Autodesk Inventor part; units mm, degrees
ref_plane "YZ Plane" through (0, 0, 0) normal (1, 0, 0) x (0, 1, 0)
ref_plane "XZ Plane" through (0, 0, 0) normal (0, 1, 0) x (-1, 0, 0)
ref_plane "XY Plane" through (0, 0, 0) normal (0, 0, 1) x (1, 0, 0)
sketch "Sketch1" plane through (0, 0, 0) normal (0, 1, 0) x (-1, 0, 0)
  arc A0 (16.9801, 0.913) -> (16.9801, -0.913) centre (-4, 0) ccw
  circle A1 centre (-4, 0) radius 21
  circle A2 centre (-4, 0) radius 19.1
  line L0 (17, 0) -> (25, 0)
  line L1 (25, 0) -> (25, -1.5)
  line L2 (25, -1.5) -> (15.041, -1.5)
  line L3 (25, 0) -> (25, 1.5)
  line L4 (25, 1.5) -> (15.041, 1.5)
  line L5 (25, -1.5) -> (25, -3)
  line L6 (25, -3) -> (14.8629, -3)
  line L7 (25, 1.5) -> (25, 3)
  line L8 (25, 3) -> (14.8629, 3)
  line L9 (-25, 0) -> (-34, 0)
  line L10 (-34, 0) -> (-42, 0)
  line L11 (-42, 0) -> (-42, 27.5)
  line L12 (-42, 27.5) -> (-34, 27.5)
  line L13 (-34, 27.5) -> (-34, 0)
  line L14 (-42, 0) -> (-42, -27.5)
  line L15 (-42, -27.5) -> (-34, -27.5)
  line L16 (-34, -27.5) -> (-34, 0)
  line L17 (-29.5, 0) -> (-29.5, 3)
  line L18 (-29.5, 3) -> (-24.7846, 3)
  line L19 (-29.5, 3) -> (-34, 3)
  line L20 (-29.5, 0) -> (-29.5, -3)
  line L21 (-29.5, -3) -> (-24.7846, -3)
  line L22 (-29.5, -3) -> (-34, -3)
  point P0 (-22.9783, -26)
  point P1 (16.7846, 3)
  point P2 (16.7846, -3)
  point P3 (-24.7846, 3)
  dimension "d8" = 38.2
  dimension "d9" = 8
  dimension "d10" = 1.5
  dimension "d11" = 1.5
  dimension "d12" = 1.5
  dimension "d13" = 1.5
  dimension "d31" = 21
  dimension "d60" = 9
  dimension "d61" = 8
  dimension "d62" = 27.5
  dimension "d63" = 27.5
  dimension "d64" = 3
  dimension "d65" = 3
extrude "Extrusion1" add sketch "Sketch1" along normal blind 23 contours A0 L8 A2 L6 | A0 L9 L17 L18 | A0 L21 L20 L9 | L8 L7 L4 A0 | A0 L4 A2 L8 | L17 L9 L13 L19 | L20 L22 L16 L9 | L13 L10 L11 L12 | L6 A2 L2 A0 | A0 L2 L5 L6 | L16 L15 L14 L10
sketch "Sketch4" plane through (-16.7846, 0, -3) normal (0, 0, -1) x (-1, 0, 0)
  line L0 (0, 0) -> (-41.5692, 0)
  line L1 (8.2154, 0) -> (8.2154, 23)
  line L2 (0, 0) -> (8.2154, 0)
  line L3 (8.2154, 0) -> (8.2154, 23)
  line L4 (8.2154, 23) -> (0, 23)
  line L5 (0, 23) -> (0, 0)
  line L6 (0, 11.5) -> (8.2154, 11.5)
  line L7 (4.1077, 11.5) -> (4.1077, 23)
  line L8 (4.1077, 11.5) -> (4.1077, 0)
  point P0 (-16.7846, 0)
  point P1 (4.1077, 5.75)
  point P2 (4.1077, 17.25)
hole "Hole2" at (-20.8923, 5.75, -3) at (-20.8923, 17.25, -3) direction (0, 0, 1) diameter 4 depth 8 tip angle 118
sketch "Sketch8" plane through (0, 23, 0) normal (0, 1, 0) x (1, 0, 0)
  line L0 (34, 3) -> (24.7846, 3)
  line L1 (34, 3) -> (24.7846, 3)
  line L2 (34, 27.5) -> (34, 3)
  line L3 (34, 3) -> (34, 27.5)
  line L4 (42, -27.5) -> (42, 27.5)
  line L5 (34, 27.5) -> (42, 27.5)
  line L6 (42, 27.5) -> (42, -27.5)
  line L7 (42, -27.5) -> (34, -27.5)
  line L8 (24.7846, -3) -> (34, -3)
  line L9 (34, -27.5) -> (34, -3)
  line L10 (34, -3) -> (24.7846, -3)
  arc A0 (24.7846, 3) -> (-16.7846, 3) centre (4, 0) ccw
  line L11 (4, 21) -> (4, 0)
  circle A1 centre (4, 0) radius 21
  point P0 (0, 0)
  point P1 (24.7846, 3)
  point P2 (24.7846, -3)
  dimension "d78" = 42
extrude "Extrusion5" cut sketch "Sketch8" against normal blind 19.5 contours L2 L5 L4 L7 L9 L8 A1 L0
sketch "Sketch9" plane through (0, 3.5, 0) normal (0, 1, 0) x (1, 0, 0)
  line L0 (34, 3) -> (34, 27.5)
  line L1 (34, -3) -> (34, 3)
  line L2 (34, 3) -> (34, 0)
  line L3 (42, 27.5) -> (42, -27.5)
  line L4 (42, 0) -> (34, 0)
  line L5 (38, 0) -> (38, -22.5)
  line L6 (38, 0) -> (38, 22.5)
  point P0 (0, 0)
  dimension "d69" = 22.5
  dimension "d70" = 22.5
hole "Hole4" at (38, 3.5, -22.5) at (38, 3.5, 22.5) direction (0, -1, 0) diameter 3 depth 8 tip angle 118
properties part number "Bracket kamera"
Verification items for the finished model (mm, model axes). A direction names the side the tool comes from. Coordinates: 2 decimals unless noted, no trailing zeros. Loops run counter-clockwise (first coordinate to the right, second up) from the corner with the lowest first, then second, coordinate; pieces in that order, holes last. Notation, with made-up numbers: (-39, -11.5) - (-31, -11.5) arc R24 cw to (-31, 7.5) - close; hole circle Ø6 at (59.25, 14.25). An arc over 180 degrees is marked (long way). Return JSON: item names as keys, results as strings.
1. Section check A-A, the plane z = -22.5. Record the boundary of the cut face in (x, y), then the cut area to 3 significant figures.
Established:
{"outline": "(34, 0) - (36.5, 0) - (36.5, 3.5) - (34, 3.5) - close; (39.5, 0) - (42, 0) - (42, 3.5) - (39.5, 3.5) - close", "area": "17.5 mm2"}
2. Section check B-B, the plane x = 38. Record the boundary of the cut face in (y, z), then the cut area to 4 significant figures.
Established:
{"outline": "(0, -27.5) - (3.5, -27.5) - (3.5, -24) - (0, -24) - close; (0, -21) - (3.5, -21) - (3.5, 21) - (0, 21) - close; (0, 24) - (3.5, 24) - (3.5, 27.5) - (0, 27.5) - close", "area": "171.5 mm2"}
3. Mould release check, pull along Z, two halves, no side actions. Record for faces 1 (the cylindrical face through (39.464, 1.726, 22.175)), 2 (the flat face through (29, 2, -3)), 3 (the cylindrical face through (-19.68, 15.66, -2.24)): +Z half, -Z half, draft (parallel to the pull), parting line (faces both ways), or undercut.
Established:
{"face 1": "undercut", "face 2": "-Z half", "face 3": "draft"}
4. Tool access check on faces 4 (the flat face through (-20, 11, 1.5)), 5 (the flat face through (29, 2, 3)), 6 (the flat face through (34, 2, -15)). Record the directions out of +Z, -Z, +X, -X, +Y, -Y that give a thin tool (end or side, any length) a straight path to the whole face; none if there is none.
Established:
{"face 4": "-X, +Y, -Y", "face 5": "+Z, +Y, -Y", "face 6": "-Z, +Y, -Y"}
5. Section check D-D, the plane z = 14. Record the boundary of the cut face in (x, y), then the cut area to 3 significant figures.
Established:
{"outline": "(-11.65, 0) - (-8.99, 0) - (-8.99, 23) - (-11.65, 23) - close; (16.99, 0) - (19.65, 0) - (19.65, 23) - (16.99, 23) - close; (34, 0) - (42, 0) - (42, 3.5) - (34, 3.5) - close", "area": "150 mm2"}
6. Go/stop test with flat-tipped pins: pin 1 (8 mm diameter, centred on y = 17, z = -20.5, fed in from -X); pin 2 (3 mm diameter, centred on x = 31.5, y = 2, fed in from +Z); pin 3 (4 mm diameter, centred on y = 1, z = 12, fed in from -X). Record where each tip stops, or that it passes through.
Established:
{"pin 1": "stops at x = -8.99", "pin 2": "stops at z = 3", "pin 3": "stops at x = -14.47"}
7. Section check C-C, the plane x = 4. Record the boundary of the cut face in (y, z).
Established:
{"outline": "(0, -21) - (23, -21) - (23, -19.1) - (0, -19.1) - close; (0, 19.1) - (23, 19.1) - (23, 21) - (0, 21) - close"}
8. Thickness scan on L1, parallel to Z at x = 38, y = 2.8; L2, parallel to X at y = 17.25, z = 2.65; L3, parallel to X at y = 7, z = -2.5. Record the ranges inside material, lowest first.
Established:
{"L1": "z = -27.5 to -24, -21 to 21, 24 to 27.5", "L2": "x = -25 to -22.89, -18.89 to -14.92, 22.92 to 24.83", "L3": "x = -25 to -22.45, -19.33 to -14.94, 22.94 to 24.85"}
